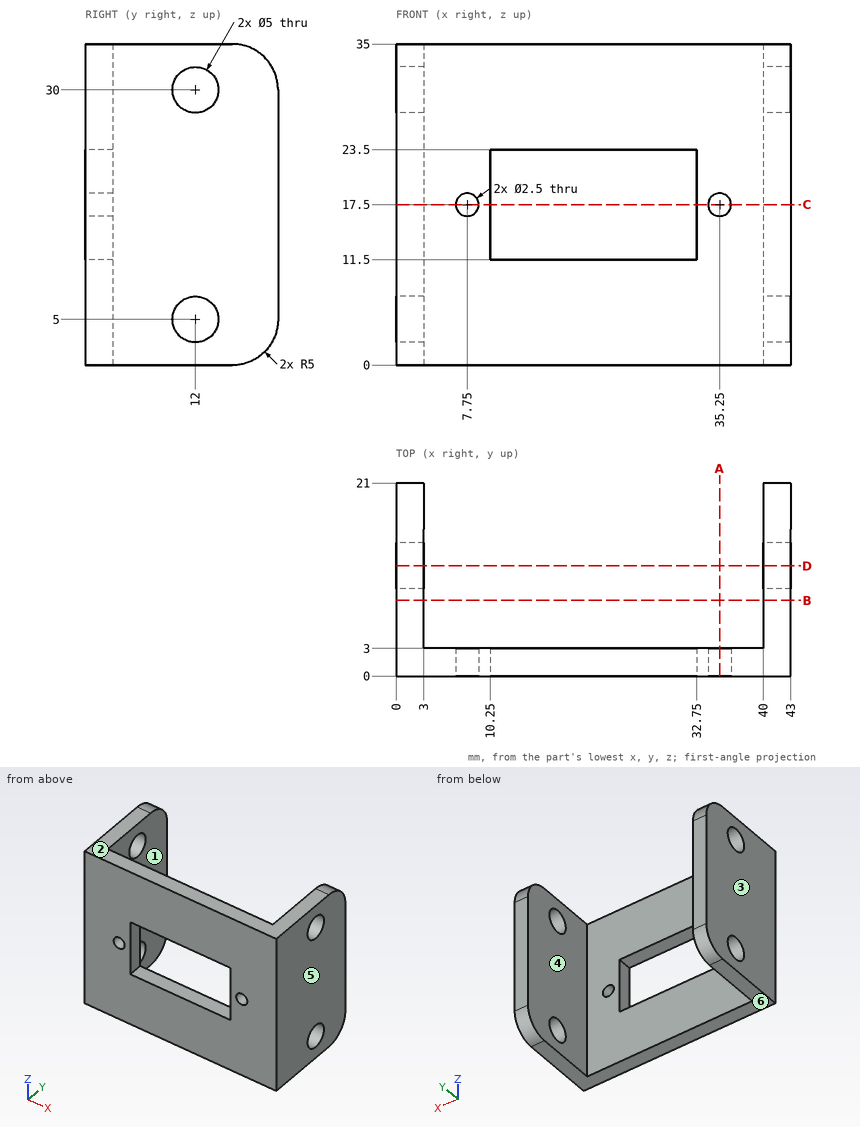
Geometry check sheet. Reference: drawing and pictorial views, mm from the part's lowest x, y, z. A direction names the side the tool comes from. Round coordinates to 2 decimals unless told otherwise and drop trailing zeros. Order: outer loops, then holes, each group sorted by start corner. A loop starts at its lowest first (then second) coordinate and runs counter-clockwise, first axis right, second up. Notation, with made-up numbers: M -14,-18.75 L -4,-18.75 A24 cw -4,15.25 Z; hole C 7.5,50 d8. An arc over 180 degrees is marked long. Answer in a Markdown table with one row per item.
(1) Sectioned sample at D-D, the plane y = 12. Record the cut outline in (x, z).
Responses:
| item | result |
|---|---|
| outline | M 0,0 L 3,0 L 3,2.5 L 0,2.5 Z; M 0,7.5 L 3,7.5 L 3,27.5 L 0,27.5 Z; M 0,32.5 L 3,32.5 L 3,35 L 0,35 Z; M 40,0 L 43,0 L 43,2.5 L 40,2.5 Z; M 40,7.5 L 43,7.5 L 43,27.5 L 40,27.5 Z; M 40,32.5 L 43,32.5 L 43,35 L 40,35 Z |
(2) Tool access check on the marked faces 1 and 2. Record the directions out of +Z, -Z, +X, -X, +Y, -Y that give a thin tool (end or side, any length) a straight path to the whole face; none if there is none.
Responses:
| item | result |
|---|---|
| face 1 | +Z, -Z, +Y |
| face 2 | +Z, +X, -X, +Y, -Y |
(3) Sectioned sample at B-B, the plane y = 8.25. Record the cut outline in (x, z).
Responses:
| item | result |
|---|---|
| outline | M 0,0 L 3,0 L 3,35 L 0,35 Z; M 40,0 L 43,0 L 43,35 L 40,35 Z |
(4) Sectioned sample at A-A, the plane x = 35.25. Record the cut outline in (y, z).
Responses:
| item | result |
|---|---|
| outline | M 0,0 L 3,0 L 3,16.25 L 0,16.25 Z; M 0,18.75 L 3,18.75 L 3,35 L 0,35 Z |
(5) Scan lines: probe 1 along X at (y, z) = (2.2, 17.5); probe 2 along Z at (x, y) = (1.5, 12); probe 3 along X at (y, z) = (5.25, 20). Record each from-to range of solid material in increasing order. Write a range as from..to.
Responses:
| item | result |
|---|---|
| probe 1 | x = 0..6.5, 9..10.25, 32.75..34, 36.5..43 |
| probe 2 | z = 0..2.5, 7.5..27.5, 32.5..35 |
| probe 3 | x = 0..3, 40..43 |
(6) Sectioned sample at C-C, the plane z = 17.5. Record the cut outline in (x, y).
Responses:
| item | result |
|---|---|
| outline | M 0,0 L 6.5,0 L 6.5,3 L 3,3 L 3,21 L 0,21 Z; M 9,0 L 10.25,0 L 10.25,3 L 9,3 Z; M 32.75,0 L 34,0 L 34,3 L 32.75,3 Z; M 36.5,0 L 43,0 L 43,21 L 40,21 L 40,3 L 36.5,3 Z |
(7) Go/stop test with a flat-tipped pin: P1, Ø10, axis at x = 17, z = 24, coming from the +Y side. Record where the tip stops, or that it passes through.
Responses:
| item | result |
|---|---|
| P1 | stops at y = 3 |
(8) Draft check along X on the marked faces 3, 4, 5 and 6. Enter one of: released by +X, released by -X, zero draft, split by the parting line, or undercut.
Responses:
| item | result |
|---|---|
| face 3 | released by -X |
| face 4 | undercut |
| face 5 | released by +X |
| face 6 | zero draft |
